from build123d import *

# Parameters (mm, degrees)
ESBO_O1_R                = 1.5
ESBO_O1_R_2              = 1.4
RESSALTO_EXTRUS_O1_DEPTH = 6.5
ESBO_O2_R                = 2.5
ESBO_O2_R_2              = 1.5
RESSALTO_EXTRUS_O2_DEPTH = 0.6
FILETE1_R                = 0.5
CHANFRO1_SIZE            = 0.3
CHANFRO1_SIZE2           = 0.091719204


with BuildPart() as part:
    # Esboço1 → Ressalto-extrusão1 (new body)
    with BuildSketch(Plane.XY):
        with Locations(Location((0, 0, 0), (0, 0, 180))):
            Circle(ESBO_O1_R)
        with Locations(Location((0, 0, 0), (0, 0, 180))):
            Circle(ESBO_O1_R_2, mode=Mode.SUBTRACT)
    extrude(amount=RESSALTO_EXTRUS_O1_DEPTH)

    # Esboço2 → Ressalto-extrusão2 (add)
    with BuildSketch(Plane(origin=(0, 0, 0), x_dir=(-1, 0, 0), z_dir=(0, 0, -1))):
        Circle(ESBO_O2_R)
        Circle(ESBO_O2_R_2, mode=Mode.SUBTRACT)
    extrude(amount=-RESSALTO_EXTRUS_O2_DEPTH)

    # Filete1
    filete1_edges = [part.edges().sort_by_distance(p)[0] for p in [
        (2.5, 0, 0),
        (1.4, 0, 0),
    ]]
    fillet(filete1_edges, radius=FILETE1_R)

    # Chanfro1
    chanfro1_edges = [part.edges().sort_by_distance(p)[0] for p in [
        (1.5, 0, 6.5),
    ]]
    chanfro1_side = [part.faces().sort_by_distance(p)[0] for p in [
        (1.5, 0, 3.55),
    ]]
    chamfer(chanfro1_edges, length=CHANFRO1_SIZE, length2=CHANFRO1_SIZE2, reference=chanfro1_side[0])


solid = part.part
Input: part model. Units: mm. Frame: model coordinates. Round coordinates to 2 decimals unless told otherwise and drop trailing zeros. Order: outer loops, then holes, each group sorted by start corner. A loop starts at its lowest first (then second) coordinate and runs counter-clockwise, first axis right, second up.
1. Cut plane C-C, the plane z = 5.25. Output: boundary loops of the cut face in (x, y).
The answers:
outline: circle Ø3 at (0, 0); hole circle Ø2.8 at (0, 0)
2. Pin query (flat end, axial travel): P1, Ø1.5, axis at y = 1, z = 1, coming from the +X side. Return the tip coordinate at first contact, or that it passes through.
The answers:
P1: stops at x = 2.47
3. Material intervals for line 1 (X direction, y = -1.25, z = 1.5); line 2 (Z direction, x = -0.1, y = -1.85); line 3 (X direction, y = 0.15, z = 0.5), sorted ascending.
The answers:
line 1: x = -0.83 to -0.63, 0.63 to 0.83
line 2: z = 0 to 0.6
line 3: x = -2.5 to -1.39, 1.39 to 2.5
